Verification items for this drawing (mm, ordinates from the low corner). A direction names the side the tool comes from. Coordinates: 2 decimals unless noted, no trailing zeros. Order: outer loops, then holes, each group sorted by start corner. A loop starts at its lowest first (then second) coordinate and runs counter-clockwise, first axis right, second up.
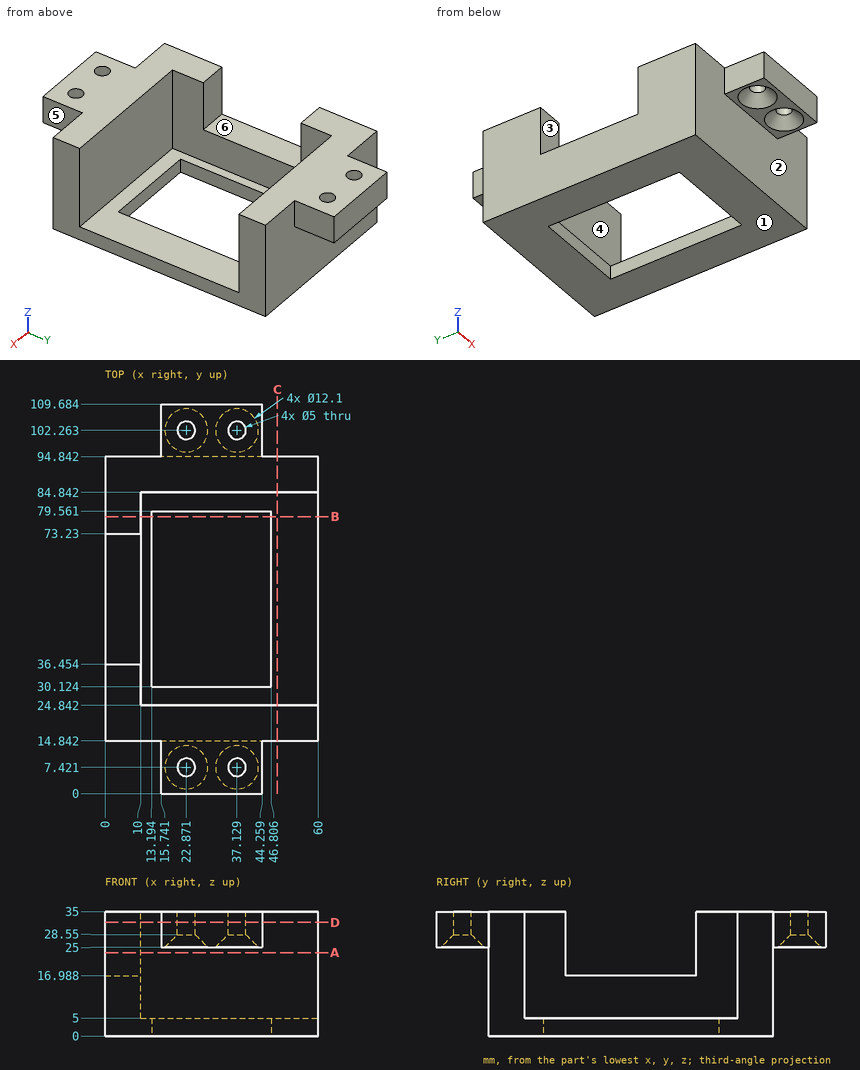
(1) Cross-section at D-D (z = 32). Enter the section's corners in (x, y) (1 decimal).
Filled in:
outline: (0, 14.8) - (15.7, 14.8) - (15.7, 0) - (44.3, 0) - (44.3, 14.8) - (60, 14.8) - (60, 24.8) - (10, 24.8) - (10, 36.5) - (0, 36.5) - close; (0, 73.2) - (10, 73.2) - (10, 84.8) - (60, 84.8) - (60, 94.8) - (44.3, 94.8) - (44.3, 109.7) - (15.7, 109.7) - (15.7, 94.8) - (0, 94.8) - close; hole circle Ø5 at (22.9, 7.4); hole circle Ø5 at (22.9, 102.3); hole circle Ø5 at (37.1, 7.4); hole circle Ø5 at (37.1, 102.3)
(2) Cross-section at A-A (z = 23.5). Enter the section's corners in (x, y) (1 decimal).
Filled in:
outline: (0, 14.8) - (60, 14.8) - (60, 24.8) - (10, 24.8) - (10, 36.5) - (0, 36.5) - close; (0, 73.2) - (10, 73.2) - (10, 84.8) - (60, 84.8) - (60, 94.8) - (0, 94.8) - close
(3) Tool access check on the marked faces 4, 5 and 6. Record the directions out of +Z, -Z, +X, -X, +Y, -Y that give a thin tool (end or side, any length) a straight path to the whole face; none if there is none.
Filled in:
face 4: +Z, +X
face 5: +Z, -Z, +X, -Y
face 6: +Z, +X, -X
(4) Release check for a two-part mould opening along Y. For the marked faces 1, 2 and 3 record: +Y half, -Y half, draft (parallel to the pull), parting line (faces both ways), or undercut.
Filled in:
face 1: draft
face 2: -Y half
face 3: undercut
(5) Thickness scan on probe 1 along Y at (x, z) = (3, 24) (1 decimal); probe 2 along Y at (x, z) = (25, 17); probe 3 along X at (y, z) = (26.5, 26.5). Record the ranges inside material, lowest first.
Filled in:
probe 1: y = 14.8 to 36.5, 73.2 to 94.8
probe 2: y = 14.84 to 24.84, 84.84 to 94.84
probe 3: x = 0 to 10
(6) Cross-section at C-C (x = 48.5). Enter the section's corners in (y, z).
Filled in:
outline: (14.84, 0) - (94.84, 0) - (94.84, 35) - (84.84, 35) - (84.84, 5) - (24.84, 5) - (24.84, 35) - (14.84, 35) - close
(7) Go/stop test with flat-tipped pins: P1, Ø6, axis at x = 32, z = 13, coming from the -Y side; P2, Ø11, axis at y = 5, z = 31.5, coming from the -X side; P3, Ø8, axis at x = 44, y = 58.5, coming from the +Z side. Record where each tip stops, or that it passes through.
Filled in:
P1: stops at y = 14.84
P2: stops at x = 15.74
P3: stops at z = 5
(8) Cross-section at B-B (y = 78). Enter the section's corners in (x, z) (1 decimal), and give its area (3 significant figures).
Filled in:
outline: (0, 0) - (13.2, 0) - (13.2, 5) - (10, 5) - (10, 35) - (0, 35) - close; (46.8, 0) - (60, 0) - (60, 5) - (46.8, 5) - close
area: 432 mm2
